Geometry: see drawing. Coordinates: mm, zero at the bounding-box minimum. Round coordinates to 2 decimals unless told otherwise and drop trailing zeros. Write each loop counter-clockwise with the first axis right and the second up, starting at its lowest first coordinate (ties: lowest second). Pieces come first, ordered by that corner, then holes. Notation, with made-up numbers: (24.5, -40) -> (83.5, -40) arc R26 cw to (83.5, -11) -> close; hole circle Ø9 at (50, -2). An arc over 180 degrees is marked (long way). Write item = value, one per line.
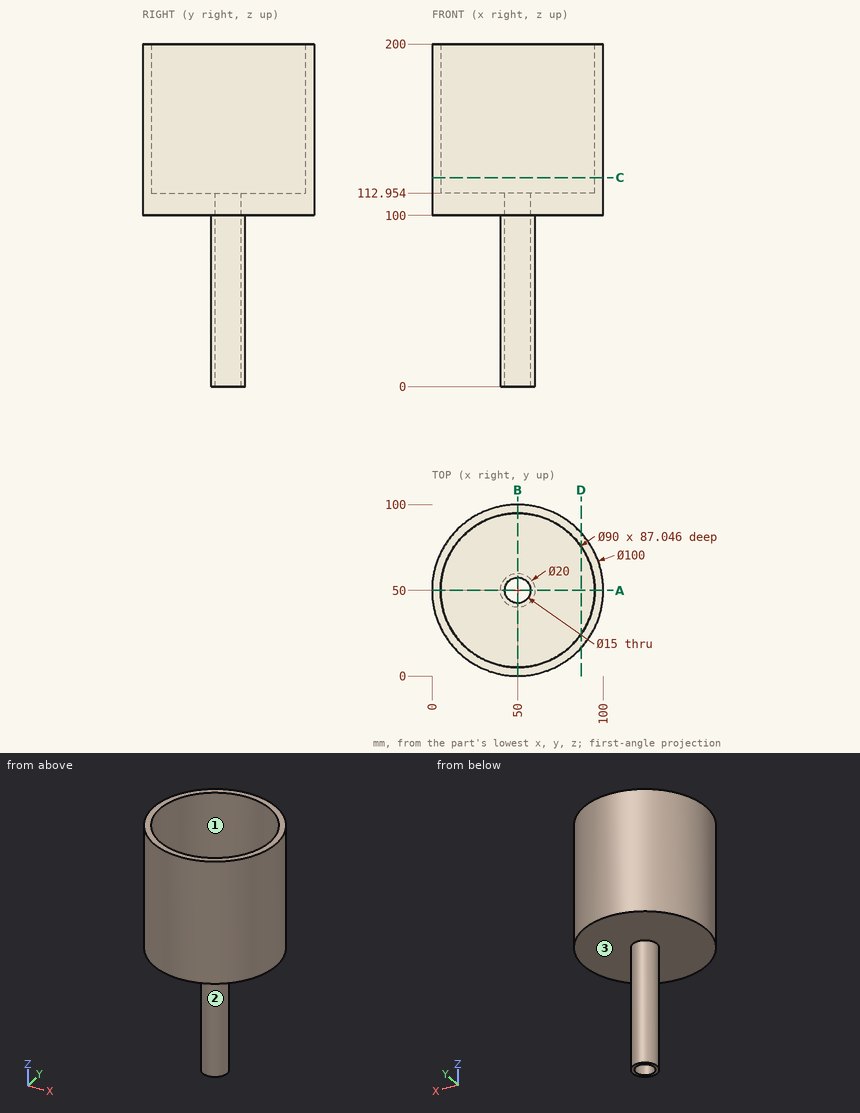
1) Cut plane C-C (z = 122). Return the cut outline in (x, y).
Solutions:
outline = circle Ø100 at (50, 50); hole circle Ø90 at (50, 50)
2) Cut plane D-D (x = 87). Return the cut outline in (y, z).
Solutions:
outline = (16.37, 100) -> (83.63, 100) -> (83.63, 200) -> (75.61, 200) -> (75.61, 112.95) -> (24.39, 112.95) -> (24.39, 200) -> (16.37, 200) -> close
3) Line query: L1, parallel to Y at x = 50, z = 143; L2, parallel to X at y = 50, z = 83; L3, parallel to Z at x = 75, y = 64.5. Output: solid intervals per line, ascending. Write a range as from..to.
Solutions:
L1 = 0..5, 95..100
L2 = 40..42.5, 57.5..60
L3 = 100..112.95
4) Cut plane A-A (y = 50). Return the cut outline in (x, z), and give its area (3 significant figures).
Solutions:
outline = (0, 100) -> (40, 100) -> (40, 0) -> (42.5, 0) -> (42.5, 112.95) -> (5, 112.95) -> (5, 200) -> (0, 200) -> close; (57.5, 0) -> (60, 0) -> (60, 100) -> (100, 100) -> (100, 200) -> (95, 200) -> (95, 112.95) -> (57.5, 112.95) -> close
area = 2,470 mm^2
5) First-contact query: P1, Ø24, axis at x = 50, y = 50, coming from the +Z side; P2, Ø3, axis at y = 29.5, z = 150, coming from the -X side; P3, Ø5, axis at x = 35.5, y = 52.5, coming from the -Z side. Flat tips, straight axial feed; report the tip coordinate or a pass-through.
Solutions:
P1 = 112.95
P2 = 3.75
P3 = 100
6) Draft query along X for the marked faces 1, 2 and 3. Return one class per face: +X half, -X half, draft (parallel to the pull), parting line (faces both ways), or undercut.
Solutions:
face_1 = undercut
face_2 = parting line
face_3 = draft
